The listing builds one solid part. Answer for the finished solid, in the listing's coordinates (mm). Give positions to 0.01 mm unless a question says otherwise; leave off trailing zeros. Loops run counter-clockwise (first coordinate to the right, second up) from the corner with the lowest first, then second, coordinate; pieces in that order, holes last. Notation, with made-up numbers: (17, -21.5) - (29, -21.5) arc R28 ccw to (29, 12.5) - close; hole circle Ø9 at (52.5, -19). An arc over 180 degrees is marked (long way). Write each question's results on one line, items separated by ' | '.
Autodesk Inventor part; units mm, degrees
ref_plane "YZ Plane" through (0, 0, 0) normal (1, 0, 0) x (0, 1, 0)
ref_plane "XZ Plane" through (0, 0, 0) normal (0, 1, 0) x (-1, 0, 0)
ref_plane "XY Plane" through (0, 0, 0) normal (0, 0, 1) x (1, 0, 0)
sketch "スケッチ1" plane through (0, 0, 0) normal (0, 1, 0) x (-1, 0, 0)
  arc A0 (139.5982, -20.0714) -> (139.3421, -16.8944) centre (139.3282, -18.4944) ccw
  arc A1 (72.9436, -26.3461) -> (139.5982, -20.0714) centre (64.9013, 416.2515) ccw
  arc A2 (54.0641, -26.1303) -> (72.9436, -26.3461) centre (67.1484, 292.5868) ccw
  arc A3 (19.3892, -19.9666) -> (54.0641, -26.1303) centre (59.4352, 104.7024) ccw
  arc A4 (-0.6275, -10.135) -> (19.3892, -19.9666) centre (42.8692, 53.13) ccw
  arc A5 (-6.31, -4.6171) -> (-0.6275, -10.135) centre (12.76, 9.3368) ccw
  arc A6 (-3.299, 4.6397) -> (-6.31, -4.6171) centre (-1.4678, -1.074) ccw
  arc A7 (5.2215, 5.7549) -> (-3.299, 4.6397) centre (4.0256, -18.2153) ccw
  arc A8 (36.4188, 0) -> (5.2215, 5.7549) centre (-0.7578, -114.096) ccw
  arc A9 (36.4188, 0) -> (38.3204, -0.6152) centre (185.125, 456.3841) ccw
  arc A10 (38.3204, -0.6152) -> (139.3421, -16.8944) centre (142.307, 323.0926) ccw
  point P0 (0, 0)
extrude "押し出し1" add sketch "スケッチ1" along normal mid plane 4
sketch "スケッチ2" plane through (0, -2, 0) normal (0, -1, 0) x (1, 0, 0)
  circle A0 centre (-6.8478, -1.4519) radius 3
  circle A1 centre (-92.934, -19.7045) radius 3
  line L0 (0, 0) -> (-112.4991, -23.8528)
  arc A2 (-139.5982, -20.0714) -> (-72.9436, -26.3461) centre (-64.9013, 416.2515) ccw
  dimension "d3" = 6
  dimension "d4" = 6
  dimension "d5" = 115
  dimension "d6" = 7
  dimension "d7" = 95
extrude "押し出し2" cut sketch "スケッチ2" against normal through all
thicken "厚み1" operation cut thickness 1 both sides no extend neighbours no toward (0.0338891, 0, -0.9994256) faces at (-130.7847, 0.6667, -16.7121) (-37.4749, 0.6667, -0.3428) (-8.7492, -0.6667, 5.5268) (2.3792, -0.6667, 4.9143) (6.574, -0.6667, -4.2247) (1.3466, -0.6667, -9.6205) (-17.0344, -0.6667, -19.1679) (-50.1454, -0.6667, -25.9105) (-56.1608, 0.6667, -26.2095) (-102.6817, 0.6667, -24.804) (-139.7269, 0.6667, -20.0439)
properties part number "flap_s" material "木材 (オーク)"
Item 1: Flat-ended cylindrical pins translate along their axes: P1, Ø8, axis at x = -6.85, z = -1.45, coming from the -Y side; P2, Ø5, axis at x = -92.93, z = -19.7, coming from the +Y side. Find the tip coordinate at first contact, or state that the pin passes through.
Values found:
P1: stops at y = -2 | P2: passes through
Item 2: For a pull along Z with two mould halves and no side action, classify faces 1 (the face through (-0.983, -0.028, 4.583)), 2 (the face through (-9.6, -0.03, -14.95)), 3 (the face through (-95.15, -0.03, -17.68)) as released by +Z, released by -Z, zero draft, split by the parting line, or undercut.
Values found:
face 1: released by +Z | face 2: released by -Z | face 3: undercut
Item 3: A cutting plane is placed at B-B, the plane x = -27.5. Determine the outline of the cut face in (y, z).
Values found:
outline: (-2, -21.26) - (2, -21.26) - (2, 1.5) - (-2, 1.5) - close
Item 4: Find the intervals of material crossed by line 1 along Z through (x, y) = (-95, 0.95); line 2 along Z through (x, y) = (-33, 1.65); line 3 along Z through (x, y) = (-58, -0.4), in increasing order. Write a range as [from, to].
Values found:
line 1: z = [-24.39, -21.88], [-17.53, -14.61] | line 2: z = [-22.52, 0.02] | line 3: z = [-25.27, -7.32]
Item 5: A cutting plane is placed at A-A, the plane y = 0.4. Determine the outline of the cut face in (x, z), plus the area to 3 significant figures.
Values found:
outline: (-139.43, -19.09) arc R441.67 ccw to (-72.93, -25.35) arc R317.97 ccw to (-54.11, -25.13) arc R129.94 ccw to (-19.7, -19.01) arc R75.78 ccw to (0.06, -9.31) arc R22.63 ccw to (5.5, -4.03) arc R5 ccw to (2.99, 3.69) arc R23 ccw to (-5.17, 4.76) arc R119 ccw to (-36.11, -0.95) arc R473.93 cw to (-38.01, -1.57) arc R341 cw to (-139.33, -17.89) arc R0.6 ccw to start; hole circle Ø6 at (-92.93, -19.7); hole circle Ø6 at (-6.85, -1.45) | area: 1,940 mm²
Item 6: A cutting plane is placed at C-C, the plane z = -12.5. Determine the outline of the cut face in (x, y), plus the area to 3 significant figures.
Values found:
outline: (-81.82, -2) - (-4.99, -2) - (-4.99, 2) - (-81.82, 2) - close | area: 307 mm²
